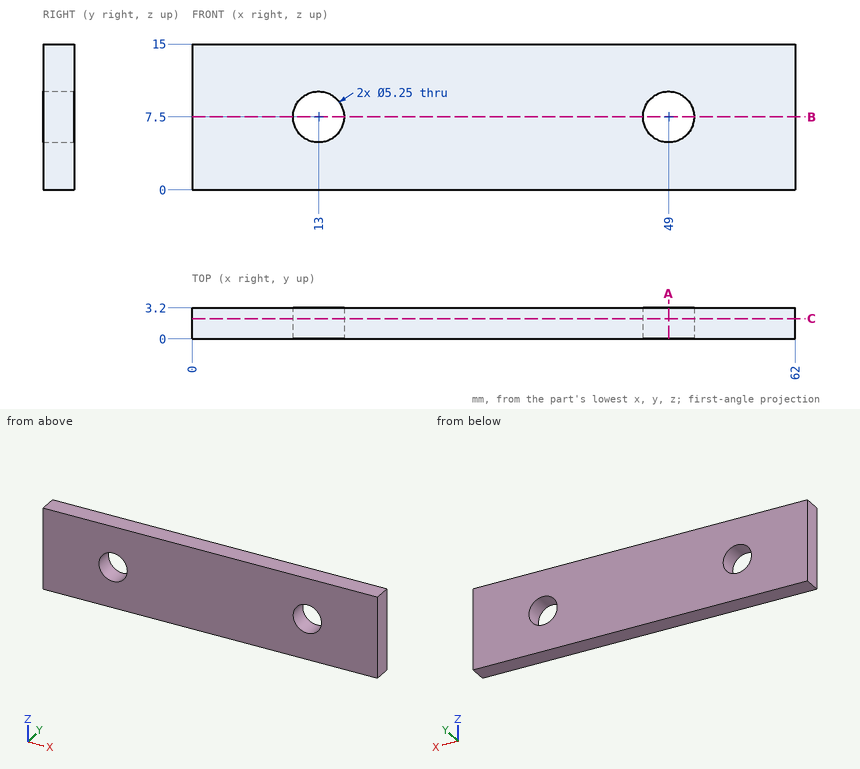
Design review of the part shown in the three views and the two pictorial views. Dimensions are in mm from the part's minimum x, y and z. Give positions to 0.01 mm unless a question says otherwise; leave off trailing zeros. Loops run counter-clockwise (first coordinate to the right, second up) from the corner with the lowest first, then second, coordinate; pieces in that order, holes last. Notation, with made-up numbers: (46, -40) -> (96, -40) arc R17 ccw to (96, -16) -> close; hole circle Ø7 at (18.5, -17.5). An arc over 180 degrees is marked (long way). Answer as a JSON object with one key per item and string values. Group by question number.
Q1. Take a section at C-C (y = 2.1). Write out the cut boundary in (x, z) (3 decimals).
Q2. Wall thickness on line 1 along X through (y, z) = (1.5, 7.75); line 2 along Z through (x, y) = (13, 2.45) (3 decimals); line 3 along X through (y, z) = (2.85, 5.5): over which ranges is each line inside the solid? List them lowest first.
Q3. Insertion check: pin 1 (4 mm diameter, centred on x = 49, z = 7.5, fed in from +Y). The pin has a flat end and moves straight along its axis. Give the tip position at first contact, or say it passes through.
Q4. Take a section at A-A (x = 49). Write out the cut boundary in (y, z) (3 decimals).
Q5. Take a section at B-B (z = 7.5). Write out the cut boundary in (x, y) (3 decimals), plus the area to 3 significant figures.
Answer below:
{
 "1": {"outline": "(0, 0) -> (62, 0) -> (62, 15) -> (0, 15) -> close; hole circle Ø5.25 at (13, 7.5); hole circle Ø5.25 at (49, 7.5)"},
 "2": {"line 1": "x = 0 to 10.39, 15.61 to 46.39, 51.61 to 62", "line 2": "z = 0 to 4.875, 10.125 to 15", "line 3": "x = 0 to 11.3, 14.7 to 47.3, 50.7 to 62"},
 "3": {"pin 1": "passes through"},
 "4": {"outline": "(0, 0) -> (3.2, 0) -> (3.2, 4.875) -> (0, 4.875) -> close; (0, 10.125) -> (3.2, 10.125) -> (3.2, 15) -> (0, 15) -> close"},
 "5": {"outline": "(0, 0) -> (10.375, 0) -> (10.375, 3.2) -> (0, 3.2) -> close; (15.625, 0) -> (46.375, 0) -> (46.375, 3.2) -> (15.625, 3.2) -> close; (51.625, 0) -> (62, 0) -> (62, 3.2) -> (51.625, 3.2) -> close", "area": "165 mm2"}
}
